from build123d import *

# Parameters (mm, degrees)
BOSS_EXTRUDE4_DEPTH = 80
BOSS_EXTRUDE5_DEPTH = 57
CUT_EXTRUDE1_DEPTH  = 3


with BuildPart() as part:
    # Sketch8 → Boss-Extrude4 (new body)
    with BuildSketch(Plane(origin=(0, 58, 0), x_dir=(1, 0, 0), z_dir=(0, 1, 0))):
        with BuildLine():
            Line((-11.242998334, -12), (11.242998334, -12))
            ThreePointArc((11.242998334, -12), (14.65898123, -10.932652517), (16.859617211, -8.110353618))
            add(Edge.make_bspline(
                [(16.859617211, -8.110353618), (17.850691543, -5.472650271), (18.834301198, 0.028433299), (17.819526576, 5.426475932), (16.811684839, 8.109721769)],
                knots=[0.167422492, 0.167422492, 0.167422492, 0.167422492, 0.502499344, 0.837905074, 0.837905074, 0.837905074, 0.837905074], degree=3))
            ThreePointArc((16.811684839, 8.109721769), (14.611088933, 10.932460371), (11.194828596, 12))
            Line((11.194828596, 12), (-11.194828596, 12))
            ThreePointArc((-11.194828596, 12), (-14.611088933, 10.932460371), (-16.811684839, 8.109721769))
            add(Edge.make_bspline(
                [(-16.859617211, -8.110353618), (-17.850691543, -5.472650271), (-18.834301198, 0.028433299), (-17.819526576, 5.426475932), (-16.811684839, 8.109721769)],
                knots=[0.167422492, 0.167422492, 0.167422492, 0.167422492, 0.502499344, 0.837905074, 0.837905074, 0.837905074, 0.837905074], degree=3))
            ThreePointArc((-16.859617211, -8.110353618), (-14.65898123, -10.932652517), (-11.242998334, -12))
        make_face()
        with BuildLine():
            Line((-13, -10), (13, -10))
            ThreePointArc((13, -10), (14.414213562, -9.414213562), (15, -8))
            Line((15, -8), (15, 8))
            ThreePointArc((15, 8), (14.414213562, 9.414213562), (13, 10))
            Line((13, 10), (-13, 10))
            ThreePointArc((-13, 10), (-14.414213562, 9.414213562), (-15, 8))
            Line((-15, 8), (-15, -8))
            ThreePointArc((-15, -8), (-14.414213562, -9.414213562), (-13, -10))
        make_face(mode=Mode.SUBTRACT)
    extrude(amount=BOSS_EXTRUDE4_DEPTH)

    # Sketch11 → Boss-Extrude5 (add)
    with BuildSketch(Plane(origin=(0, 58, 0), x_dir=(1, 0, 0), z_dir=(0, 1, 0))):
        with BuildLine():
            Line((13, 10), (15, 10))
            Line((15, 10), (15, 6.937911183))
            Line((15, 6.937911183), (13.5, 6.937911183))
            ThreePointArc((13.5, 6.937911183), (13.146446609, 7.084357793), (13, 7.437911183))
            Line((13, 7.437911183), (13, 10))
        make_face()
        with BuildLine():
            Line((-13, 7.437911183), (-13, 10))
            Line((-13, 10), (-15, 10))
            Line((-15, 10), (-15, 6.937911183))
            Line((-15, 6.937911183), (-13.5, 6.937911183))
            ThreePointArc((-13.5, 6.937911183), (-13.146446609, 7.084357793), (-13, 7.437911183))
        make_face()
    extrude(amount=BOSS_EXTRUDE5_DEPTH)

    # Sketch12 → Cut-Extrude1 (cut)
    with BuildSketch(Plane.XY.offset(12)):
        with BuildLine():
            Line((7.476357736, 134.986611492), (7.476357736, 114.986611492))
            ThreePointArc((7.476357736, 114.986611492), (-0.023642264, 107.486611492), (-7.523642264, 114.986611492))
            Line((-7.523642264, 114.986611492), (-7.523642264, 134.986611492))
            Line((-7.523642264, 134.986611492), (-8.023642264, 134.986611492))
            Line((-8.023642264, 134.986611492), (-8.023642264, 114.986611492))
            ThreePointArc((-8.023642264, 114.986611492), (-0.023642264, 106.986611492), (7.976357736, 114.986611492))
            Line((7.976357736, 114.986611492), (7.976357736, 134.986611492))
            Line((7.976357736, 134.986611492), (7.476357736, 134.986611492))
        make_face()
    extrude(amount=-CUT_EXTRUDE1_DEPTH, mode=Mode.SUBTRACT)


solid = part.part
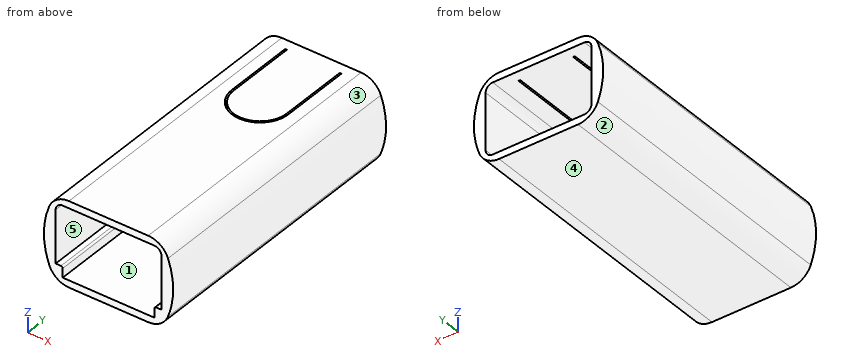
Build history of the part. All positions in model axes, mm. Face numbers are marked on the shaded views. A direction names the side the tool comes from. Coordinates: 2 decimals unless noted, no trailing zeros. Write each loop counter-clockwise with the first axis right and the second up, starting at its lowest first coordinate (ties: lowest second). Pieces come first, ordered by that corner, then holes.
(1) Cut at A-A on x = -9. List the corners of the cut face in (y, z), and give its area (3 significant figures).
(2) Pin check, flat tips, straight feed: pin 1 Ø2 at (y, z) = (120.5, 10.5) entering from -X; pin 2 Ø2 at (y, z) = (128.5, 10.5) entering from +X; pin 3 Ø12 at (y, z) = (126.5, -9) entering from +X. Stop position of each tip, or through.
(3) Cut at B-B on z = -9. List the corners of the cut face in (x, y).
(4) 3-axis set-ups, long thin cutter, end or side, ignore diameter. For the marked faces 1 and 2: which of +Z, -Z, +X, -X, +Y, -Y reach the whole face in a straight line?
(5) Mould opens along X. For the marked faces 3, 4 and 5 say: pulls with the +X half, pulls with the -X half, needs draft (parallel to the pull), parting line crosses it, or undercut.
(6) Cut at D-D on x = 2. List the corners of the cut face in (y, z).
(7) Drill centre lines: line 1 (Z direction, x = 3, y = 85); line 2 (X direction, y = 112, z = 10.25); line 3 (X direction, y = 64, z = -0.25). Where is each one in solid material? Low to high.
(8) Cut at C-C on x = -5. List the corners of the cut face in (y, z).
Working result:
1. outline: (58, -12) - (138, -12) - (138, -10) - (58, -10) - close; (58, 10) - (138, 10) - (138, 12) - (58, 12) - close
1. area: 320 mm2
2. pin 1: stops at x = -16.12
2. pin 2: stops at x = 16.12
2. pin 3: stops at x = 18.12
3. outline: (-16.39, 58) - (-13, 58) - (-13, 115) - (-14.73, 115) - (-14.73, 138) - (-16.39, 138) - close; (13, 58) - (16.39, 58) - (16.39, 138) - (14.73, 138) - (14.73, 115) - (13, 115) - close
4. face 1: +Y, -Y
4. face 2: -Z, -X, +Y, -Y
5. face 3: pulls with the +X half
5. face 4: needs draft
5. face 5: undercut
6. outline: (58, -12) - (138, -12) - (138, -10) - (58, -10) - close; (58, 10) - (107.25, 10) - (107.25, 12) - (58, 12) - close; (107.76, 10) - (138, 10) - (138, 12) - (107.76, 12) - close
7. line 1: z = -12 to -10, 10 to 12
7. line 2: x = -15.48 to -7.45, -6.9 to 6.86, 7.4 to 15.48
7. line 3: x = -18.33 to -15, 15 to 18.33
8. outline: (58, -12) - (138, -12) - (138, -10) - (58, -10) - close; (58, 10) - (108.72, 10) - (108.72, 12) - (58, 12) - close; (109.38, 10) - (138, 10) - (138, 12) - (109.38, 12) - close
